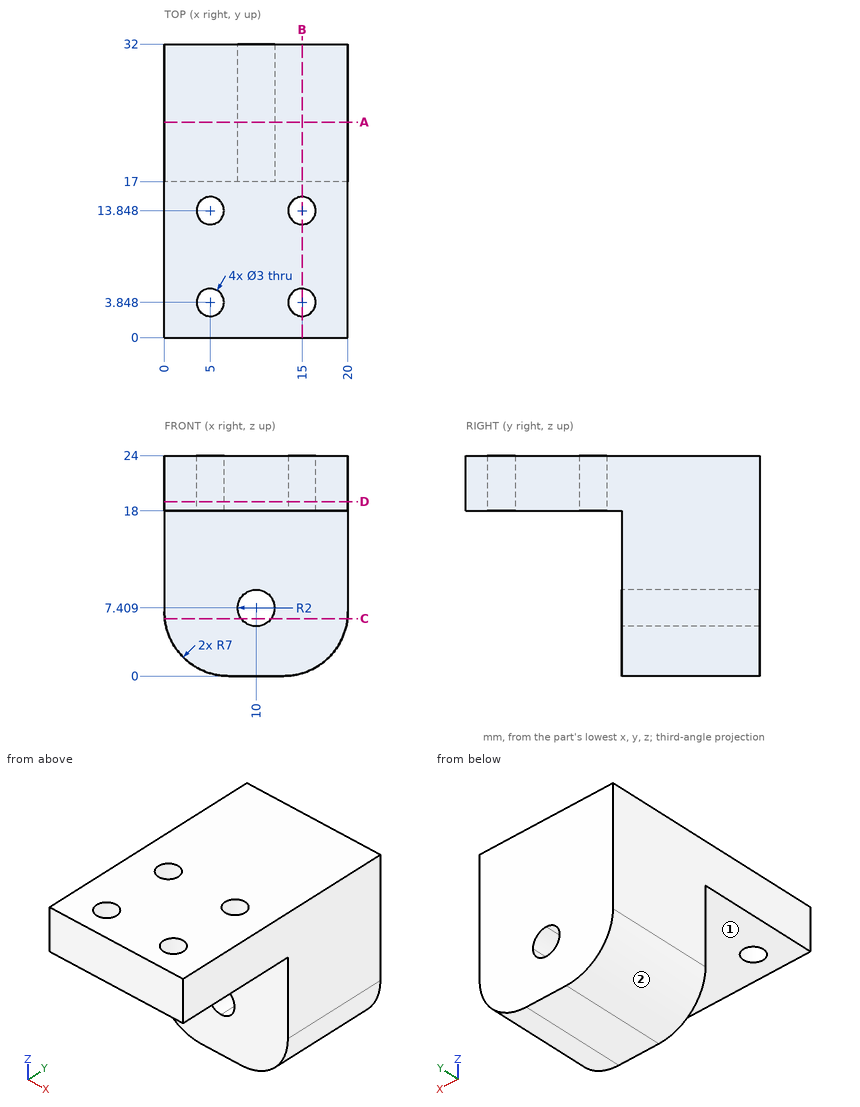
Could you check a few things on this drawing? It's one solid part, dimensions in mm from its lowest x, y, z. A direction names the side the tool comes from. Round coordinates to 2 decimals unless told otherwise and drop trailing zeros. Loops run counter-clockwise (first coordinate to the right, second up) from the corner with the lowest first, then second, coordinate; pieces in that order, holes last. Notation, with made-up numbers: M -7,70 L 46,70 A17 ccw 46,92 Z; hole C 66,63 d1. An arc over 180 degrees is marked long. Write each question's results on one line, items separated by ' | '. Start each with the question number.
(1) I want a section at B-B (x = 15). Please give me the cut outline in (y, z), then the cut area to 3 significant figures.
(2) If I drill on probe 1 along Y at (x, z) = (15, 20.8); probe 2 along Y at (x, z) = (3, 8); probe 3 along Z at (x, y) = (10.5, 7.5), over which ranges is the centre line in solid material (lowest first)? Write a range as from..to.
(3) Will these pins go through, and if not, where does the flat tip stop? P1, Ø5, axis at y = 24.5, z = 9.5, coming from the -X side; P2, Ø2, axis at x = 4.5, y = 19, coming from the -Z side; P3, Ø2.5, axis at x = 15, y = 13.85, coming from the +Z side; P4, Ø4, axis at x = 6.5, z = 3, coming from the -Y side.
(4) I want a section at A-A (y = 23.5). Please give me the cut outline in (x, z).
(5) I want a section at D-D (z = 19). Please give me the cut outline in (x, y).
(6) I want a section at C-C (z = 6.25). Please give me the cut outline in (x, y), then the cut area to 3 significant figures.
(7) On a 3-axis mill with a long thin cutter (end or side, diameter ignored), from which of +Z, -Z, +X, -X, +Y, -Y can I reach the whole of each face in a straight line? I mean the marked faces 1 and 2. Say none if no direction works.
Solved:
1) outline: M 0,18 L 2.35,18 L 2.35,24 L 0,24 Z; M 5.35,18 L 12.35,18 L 12.35,24 L 5.35,24 Z; M 15.35,18 L 17,18 L 17,0.29 L 32,0.29 L 32,24 L 15.35,24 Z | area: 422 mm²
2) probe 1: y = 0..2.35, 5.35..12.35, 15.35..32 | probe 2: y = 17..32 | probe 3: z = 18..24
3) P1: stops at x = 0 | P2: stops at z = 0.16 | P3: passes through | P4: stops at y = 17
4) outline: M 0,7 A7 ccw 7,0 L 13,0 A7 ccw 20,7 L 20,24 L 0,24 Z; hole C 10,7.41 d4
5) outline: M 0,0 L 20,0 L 20,32 L 0,32 Z; hole C 5,3.85 d3; hole C 5,13.85 d3; hole C 15,3.85 d3; hole C 15,13.85 d3
6) outline: M 0.04,17 L 8.37,17 L 8.37,32 L 0.04,32 Z; M 11.63,17 L 19.96,17 L 19.96,32 L 11.63,32 Z | area: 250 mm²
7) face 1: -Z, +X, -X, -Y | face 2: -Z, -X, +Y, -Y
